```python
from build123d import *

# Parameters (mm, degrees)
SKETCH1_R           = 2.5
BOSS_EXTRUDE1_DEPTH = 67.21
SKETCH2_R           = 3.5
BOSS_EXTRUDE2_DEPTH = 2
CHAMFER1_SIZE       = 1
SKETCH3_R           = 1.5
CUT_EXTRUDE1_DEPTH  = 5


with BuildPart() as part:
    # Sketch1 → Boss-Extrude1 (new body)
    with BuildSketch(Plane(origin=(0, 0, 0), x_dir=(1, 0, 0), z_dir=(0, 1, 0))):
        Circle(SKETCH1_R)
    extrude(amount=BOSS_EXTRUDE1_DEPTH)

    # Sketch2 → Boss-Extrude2 (add)
    with BuildSketch(Plane(origin=(0, 67.21, 0), x_dir=(1, 0, 0), z_dir=(0, 1, 0))):
        Circle(SKETCH2_R)
    extrude(amount=BOSS_EXTRUDE2_DEPTH)

    # Chamfer1
    chamfer1_edges = [part.edges().sort_by_distance(p)[0] for p in [
        (-3.5, 69.21, 0),
    ]]
    chamfer(chamfer1_edges, length=CHAMFER1_SIZE)

    # Sketch3 → Cut-Extrude1 (cut)
    with BuildSketch(Plane.XZ):
        Circle(SKETCH3_R)
    extrude(amount=-CUT_EXTRUDE1_DEPTH, mode=Mode.SUBTRACT)


solid = part.part
```
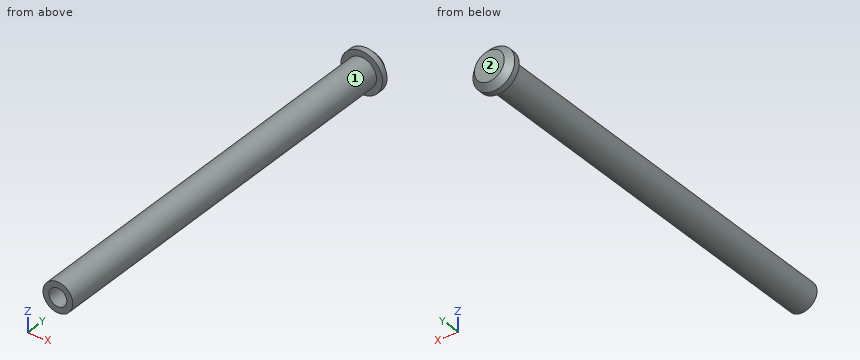
Source: CAD feature listing. Evaluate the final solid. Frame: model axes, mm. Face numbers are marked on the shaded views. A direction names the side the tool comes from. Give positions to 0.01 mm unless a question says otherwise; leave off trailing zeros. Order: outer loops, then holes, each group sorted by start corner. A loop starts at its lowest first (then second) coordinate and runs counter-clockwise, first axis right, second up.
(1) Section query A-A (z = 0). Return the cut outline in (x, y), plus the area to 3 significant figures.
(2) Contact query for flat-ended pins moving along their axis: P1, Ø0.9, axis at x = 0.5, z = 0.5, coming from the -Y side; P2, Ø2, axis at y = 59, z = -2.5, coming from the +X side; P3, Ø2, axis at y = 13, z = 1.5, coming from the -X side. Output: stop coordinate, or through.
(3) Access query for the marked faces 1 and 2. Directions: +Z, -Z, +X, -X, +Y, -Y. A direction counts if a zero-diameter tool reaches every point of the face in a straight line with its end or side. Return the directions, or none.
(4) Section query B-B (x = 0). Return the cut outline in (y, z).
(5) Section query C-C (y = 13.5). Return the cut outline in (x, z), plus the area to 3 significant figures.
(6) Material intervals for line 1 along Z through (x, y) = (0, 1.7); line 2 along Z through (x, y) = (0.25, 48); line 3 along Y through (x, z) = (-0.5, 1), sorted ascending.
Outcome:
1. outline: (-3.5, 67.21) - (-2.5, 67.21) - (-2.5, 0) - (-1.5, 0) - (-1.5, 5) - (1.5, 5) - (1.5, 0) - (2.5, 0) - (2.5, 67.21) - (3.5, 67.21) - (3.5, 68.21) - (2.5, 69.21) - (-2.5, 69.21) - (-3.5, 68.21) - close
1. area: 334 mm2
2. P1: stops at y = 5
2. P2: stops at x = 2
2. P3: stops at x = -2.45
3. face 1: -Y
3. face 2: +Z, -Z, +X, -X, +Y
4. outline: (0, -2.5) - (67.21, -2.5) - (67.21, -3.5) - (68.21, -3.5) - (69.21, -2.5) - (69.21, 2.5) - (68.21, 3.5) - (67.21, 3.5) - (67.21, 2.5) - (0, 2.5) - (0, 1.5) - (5, 1.5) - (5, -1.5) - (0, -1.5) - close
5. outline: circle Ø5 at (0, 0)
5. area: 19.6 mm2
6. line 1: z = -2.5 to -1.5, 1.5 to 2.5
6. line 2: z = -2.49 to 2.49
6. line 3: y = 5 to 69.21
